Build history of the part. All positions in model axes, mm. Round coordinates to 2 decimals unless told otherwise and drop trailing zeros. Write each loop counter-clockwise with the first axis right and the second up, starting at its lowest first coordinate (ties: lowest second). Pieces come first, ordered by that corner, then holes.
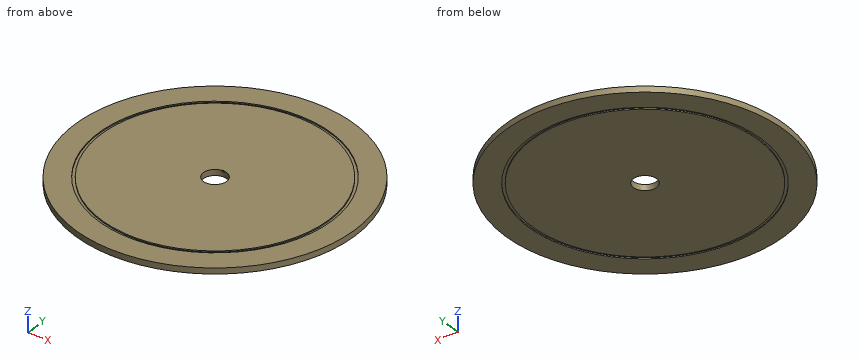
Autodesk Inventor part; units mm, degrees
ref_plane "YZ Plane" through (0, 0, 0) normal (1, 0, 0) x (0, 1, 0)
ref_plane "XZ Plane" through (0, 0, 0) normal (0, 1, 0) x (-1, 0, 0)
ref_plane "XY Plane" through (0, 0, 0) normal (0, 0, 1) x (1, 0, 0)
sketch "Sketch1" plane through (0, 0, 0) normal (0, 0, 1) x (1, 0, 0)
  circle A0 centre (0, 0) radius 152.4
  circle A1 centre (0, 0) radius 12.7
  dimension "d0" = 304.8
  dimension "d1" = 25.4
extrude "Extrusion1" add sketch "Sketch1" along normal blind 6.35
sketch "Sketch2" plane through (0, 0, 6.35) normal (0, 0, 1) x (1, 0, 0)
  point P0 (0, 0)
sketch "Sketch3" plane through (0, 0, 6.35) normal (0, 0, 1) x (1, 0, 0)
  circle A0 centre (0, 0) radius 127
  circle A1 centre (0, 0) radius 123.825
  dimension "d4" = 254
  dimension "d5" = 247.65
extrude "Extrusion2" cut sketch "Sketch3" against normal blind 1.27
sketch "Sketch4" plane through (0, 0, 0) normal (0, 0, -1) x (-1, 0, 0)
  circle A0 centre (0, 0) radius 152.4
  circle A1 centre (0, 0) radius 127
  circle A2 centre (0, 0) radius 123.825
  dimension "d8" = 254
  dimension "d9" = 247.65
extrude "Extrusion3" cut sketch "Sketch4" against normal blind 1.27 contours A1
sketch "Sketch5" plane through (0, 0, 6.35) normal (0, 0, 1) x (1, 0, 0)
  circle A0 centre (0, 0) radius 12.7
  line L0 (0, 12.7) -> (0, 13.208)
  line L1 (0, 13.208) -> (1.27, 13.208)
  line L2 (0, 13.208) -> (-1.27, 13.208)
  line L3 (-1.27, 13.208) -> (-1.27, 12.2678)
  line L4 (1.27, 13.208) -> (1.27, 12.2294)
  arc A1 (1.27, 12.6363) -> (-1.27, 12.6363) centre (0, 0) ccw
  dimension "d12" = 0.508
  dimension "d15" = 1.27
  dimension "d16" = 1.27
extrude "Extrusion4" cut sketch "Sketch5" against normal blind 1.27 contours A0 L0 L1 L4 | L3 L2 L0 A0
properties part number "PlateCenter"
1) Slice it at C-C (x = 62). Write the cut outline in (y, z), plus the area to 3 significant figures.
Results:
outline: (-139.22, 0) - (-110.84, 0) - (-110.84, 1.27) - (-107.19, 1.27) - (-107.19, 0) - (107.19, 0) - (107.19, 1.27) - (110.84, 1.27) - (110.84, 0) - (139.22, 0) - (139.22, 6.35) - (110.84, 6.35) - (110.84, 5.08) - (107.19, 5.08) - (107.19, 6.35) - (-107.19, 6.35) - (-107.19, 5.08) - (-110.84, 5.08) - (-110.84, 6.35) - (-139.22, 6.35) - close
area: 1,750 mm2
2) Slice it at B-B (z = 4). Write the cut outline in (x, y).
Results:
outline: circle Ø304.8 at (0, 0); hole circle Ø25.4 at (0, 0)
3) Wall check: L1, parallel to Y at x = 0, z = 0.75 (3 decimals); L2, parallel to Y at x = 0, z = 6 (3 decimals); L3, parallel to Y at x = -52, z = 0.75. Give the ranges that are in metal, low to high.
Results:
L1: y = -152.4 to -127, -123.825 to -12.7, 12.7 to 123.825, 127 to 152.4
L2: y = -152.4 to -127, -123.825 to -12.7, 13.208 to 123.825, 127 to 152.4
L3: y = -143.25 to -115.87, -112.38 to 112.38, 115.87 to 143.25
4) Slice it at D-D (y = 97.5). Write the cut outline in (x, z), plus the area to 3 significant figures.
Results:
outline: (-117.13, 0) - (-81.38, 0) - (-81.38, 1.27) - (-76.33, 1.27) - (-76.33, 0) - (76.33, 0) - (76.33, 1.27) - (81.38, 1.27) - (81.38, 0) - (117.13, 0) - (117.13, 6.35) - (81.38, 6.35) - (81.38, 5.08) - (76.33, 5.08) - (76.33, 6.35) - (-76.33, 6.35) - (-76.33, 5.08) - (-81.38, 5.08) - (-81.38, 6.35) - (-117.13, 6.35) - close
area: 1,460 mm2
5) Slice it at A-A (y = 0). Write the cut outline in (x, z) (3 decimals), plus the area to 3 significant figures.
Results:
outline: (-152.4, 0) - (-127, 0) - (-127, 1.27) - (-123.825, 1.27) - (-123.825, 0) - (-12.7, 0) - (-12.7, 6.35) - (-123.825, 6.35) - (-123.825, 5.08) - (-127, 5.08) - (-127, 6.35) - (-152.4, 6.35) - close; (12.7, 0) - (123.825, 0) - (123.825, 1.27) - (127, 1.27) - (127, 0) - (152.4, 0) - (152.4, 6.35) - (127, 6.35) - (127, 5.08) - (123.825, 5.08) - (123.825, 6.35) - (12.7, 6.35) - close
area: 1,760 mm2
6) Pin check, flat tips, straight feed: pin 1 Ø2 at (x, z) = (101, 3.5) entering from -Y; pin 2 Ø1 at (y, z) = (69, 2) entering from -X; pin 3 Ø3 at (x, z) = (64, 3) entering from -Y. Stop position of each tip, or through.
Results:
pin 1: stops at y = -115
pin 2: stops at x = -136.14
pin 3: stops at y = -138.99
